Geometry check sheet. Reference: drawing and pictorial views, mm from the part's lowest x, y, z. A direction names the side the tool comes from. Give positions to 0.01 mm unless a question says otherwise; leave off trailing zeros. Loops run counter-clockwise (first coordinate to the right, second up) from the corner with the lowest first, then second, coordinate; pieces in that order, holes last. Notation, with made-up numbers: M -22.5,-7.5 L 22.5,-7.5 A16 cw 22.5,22.5 Z; hole C 54.25,-13 d6. An arc over 180 degrees is marked long. One line per question, with ' | ' between items. Start each with the question number.
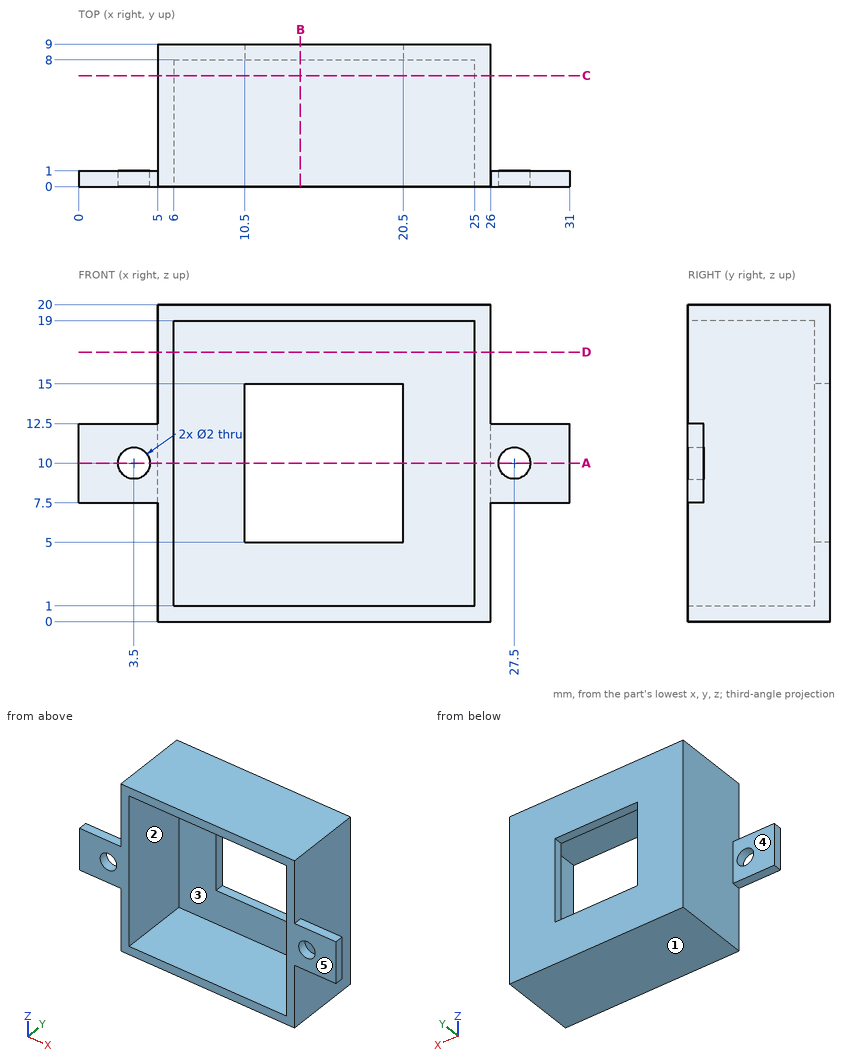
Q1. Access from +Z, -Z, +X, -X, +Y, -Y to the whole of each face (thin tool, end or side, straight path). Record for the marked faces 3, 4 and 5.
Q2. Depth check by flat-ended pin: P1, Ø0.8, axis at x = 3.5, y = 0.5, coming from the +Z side; P2, Ø0.8, axis at x = 28, y = 0.5, coming from the -Z side; P3, Ø9, axis at x = 18.5, z = 10, coming from the -Y side; P4, Ø3, axis at x = 28, z = 15, coming from the +Y side. Enter the tip coordinate at first touch or a pass-through.
Q3. Cross-section at A-A (z = 10). Record the cut outline in (x, y).
Q4. Cross-section at C-C (y = 7). Record the cut outline in (x, z).
Q5. Draft check along X on the marked faces 1 and 2. Enter one of: released by +X, released by -X, zero draft, split by the parting line, or undercut.
Q6. Cross-section at B-B (x = 14). Record the cut outline in (y, z), and give its area (3 significant figures).
Q7. Cross-section at D-D (z = 17). Record the cut outline in (x, y), and give its area (3 significant figures).
Q8. Material ranges on probe 1 along X at (y, z) = (7, 8.5); probe 2 along Z at (x, y) = (3.5, 0.5); probe 3 along Z at (x, y) = (9, 2.25), recorded low to high. Write a range as from..to.
Solved:
1) face 3: -Y | face 4: +Z, -Z, -X, +Y | face 5: +Z, -Z, +X, -X, -Y
2) P1: stops at z = 12.5 | P2: stops at z = 7.5 | P3: stops at y = 8 | P4: passes through
3) outline: M 0,0 L 2.5,0 L 2.5,1 L 0,1 Z; M 4.5,0 L 6,0 L 6,8 L 10.5,8 L 10.5,9 L 5,9 L 5,1 L 4.5,1 Z; M 20.5,8 L 25,8 L 25,0 L 26.5,0 L 26.5,1 L 26,1 L 26,9 L 20.5,9 Z; M 28.5,0 L 31,0 L 31,1 L 28.5,1 Z
4) outline: M 5,0 L 26,0 L 26,20 L 5,20 Z; hole M 6,1 L 25,1 L 25,19 L 6,19 Z
5) face 1: zero draft | face 2: undercut
6) outline: M 0,0 L 9,0 L 9,5 L 8,5 L 8,1 L 0,1 Z; M 0,19 L 8,19 L 8,15 L 9,15 L 9,20 L 0,20 Z | area: 26.0 mm²
7) outline: M 5,0 L 6,0 L 6,8 L 25,8 L 25,0 L 26,0 L 26,9 L 5,9 Z | area: 37.0 mm²
8) probe 1: x = 5..6, 25..26 | probe 2: z = 7.5..9, 11..12.5 | probe 3: z = 0..1, 19..20
